Geometry: final body of the model. Coordinates: model frame, mm. Give positions to 0.01 mm unless a question says otherwise; leave off trailing zeros. Order: outer loops, then holes, each group sorted by start corner. A loop starts at its lowest first (then second) coordinate and runs counter-clockwise, first axis right, second up. Notation, with made-up numbers: (81, -32.75) -> (111, -32.75) arc R4 cw to (111, -25.75) -> close; hole circle Ø3 at (49, -37). An arc over 180 degrees is marked (long way). Answer in a Markdown table with one row per item. Add a question column.
Q1. Line query: line 1 along X through (y, z) = (17, 5); line 2 along Y through (x, z) = (75, 6); line 3 along Y through (x, z) = (70, 5.5). Output: solid intervals per line, ascending. Write a range as from..to.
Q2. Cut plane A-A on x = -75. Return the cut outline in (y, z), and give its area (3 significant figures).
Q3. Contact query for flat-ended pins moving along their axis: P1, Ø2, axis at y = 23.5, z = 6, coming from the +X side; P2, Ø1, axis at y = -10.5, z = 6, coming from the -X side; P3, Ø4, axis at y = -3.5, z = 3, coming from the -X side. Output: stop coordinate, or through.
Q4. Cut plane D-D on z = 4.25. Count the separate pieces of the cut face and the enclosed holes in it, and give its area (3 significant figures).
Q5. Cut plane C-C on y = -19. Return the cut outline in (x, z).
Q6. Cut plane B-B on y = 63. Return the cut outline in (x, z).
from build123d import *

# Parameters (mm, degrees)
BOSS_EXTRUDE1_DEPTH  = 8
M4_CLEARANCE_HOLE1_D = 4.3
M5_CLEARANCE_HOLE1_D = 5.3


with BuildPart() as part:
    # Sketch1 → Boss-Extrude1 (new body)
    with BuildSketch(Plane.XY):
        Polygon((-82.5, 37.5), (-45, 0), (-82.5, -37.5), (-82.5, -82.5), (-37.5, -82.5), (0, -45), (37.5, -82.5), (82.5, -82.5), (82.5, -37.5), (45, 0), (82.5, 37.5), (82.5, 82.5), (37.5, 82.5), (0, 45), (-37.5, 82.5), (-82.5, 82.5), align=None)
    extrude(amount=BOSS_EXTRUDE1_DEPTH)

    # M4 Clearance Hole1 (through all)
    with Locations(Plane.XY.offset(8)):
        with Locations((-75, 76), (-45, 76), (-45, 44), (-75, 44), (-75, -44), (-45, -44), (-45, -76), (-75, -76), (75, -76), (45, -76), (45, -44), (75, -44), (75, 44), (45, 44), (45, 76), (75, 76)):
            Hole(M4_CLEARANCE_HOLE1_D / 2)

    # M5 Clearance Hole1 (through all)
    with Locations(Plane.XY.offset(8)):
        with Locations((-11, 19), (-11, -19), (11, -19), (11, 19)):
            Hole(M5_CLEARANCE_HOLE1_D / 2)


solid = part.part
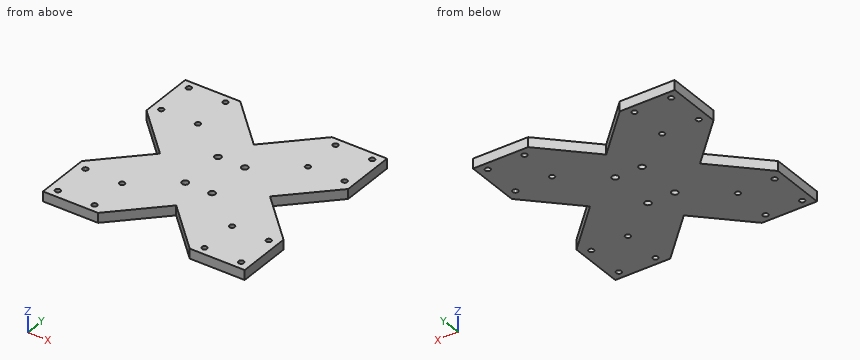
Completed:
| question | item | result |
|---|---|---|
| 1 | line 1 | x = -62..-12.74, -9.26..9.26, 12.74..62 |
| 1 | line 2 | y = -82.5..-78.15, -73.85..-46.15, -41.85..-30, 30..41.85, 46.15..73.85, 78.15..82.5 |
| 1 | line 3 | y = -82.5..-25, 25..82.5 |
| 2 | outline | (-82.5, 0) -> (-78.15, 0) -> (-78.15, 8) -> (-82.5, 8) -> close; (-73.85, 0) -> (-46.15, 0) -> (-46.15, 8) -> (-73.85, 8) -> close; (-41.85, 0) -> (-30, 0) -> (-30, 8) -> (-41.85, 8) -> close; (30, 0) -> (41.85, 0) -> (41.85, 8) -> (30, 8) -> close; (46.15, 0) -> (73.85, 0) -> (73.85, 8) -> (46.15, 8) -> close; (78.15, 0) -> (82.5, 0) -> (82.5, 8) -> (78.15, 8) -> close |
| 2 | area | 702 mm² |
| 3 | P1 | stops at x = 69.5 |
| 3 | P2 | stops at x = -56 |
| 3 | P3 | stops at x = -50.5 |
| 4 | separate pieces | 1 |
| 4 | enclosed holes | 20 |
| 4 | area | 21,300 mm² |
| 5 | outline | (-64, 0) -> (-13.65, 0) -> (-13.65, 8) -> (-64, 8) -> close; (-8.35, 0) -> (8.35, 0) -> (8.35, 8) -> (-8.35, 8) -> close; (13.65, 0) -> (64, 0) -> (64, 8) -> (13.65, 8) -> close |
| 6 | outline | (-82.5, 0) -> (-18, 0) -> (-18, 8) -> (-82.5, 8) -> close; (18, 0) -> (82.5, 0) -> (82.5, 8) -> (18, 8) -> close |
